Autodesk Inventor part; units mm, degrees
ref_plane "YZ Plane" through (0, 0, 0) normal (1, 0, 0) x (0, 1, 0)
ref_plane "XZ Plane" through (0, 0, 0) normal (0, 1, 0) x (-1, 0, 0)
ref_plane "XY Plane" through (0, 0, 0) normal (0, 0, 1) x (1, 0, 0)
sketch "スケッチ1" plane through (0, 0, 0) normal (0, 1, 0) x (-1, 0, 0)
  line L0 (0, 0) -> (-1.1547, 0)
  line L1 (-2.6, 1.05) -> (-3.5, 1.05)
  line L2 (-3.5, 1.05) -> (-3.5, 1.65)
  line L3 (-3.5, 1.65) -> (-1.5, 1.65)
  line L4 (-1.5, 1.65) -> (-1.5, 7.65)
  line L5 (-1.5, 7.65) -> (0, 7.65)
  line L6 (0, 7.65) -> (0, 0)
  arc A0 (-2.6, 1.05) -> (-1.1547, 0) centre (-1.1547, 1.5197) ccw
  dimension "d0" = 5.2
  dimension "d1" = 7
  dimension "d3" = 1.65
  dimension "d4" = 0.6
  dimension "d5" = 2.3094
  dimension "d6" = 6
  dimension "d7" = 3
revolve "回転1" add sketch "スケッチ1" angle 360 about axis through (0, 0, 7.65) along (0, 0, -1)
thread "ねじ1"
sketch "スケッチ2" plane through (0, 0, 0) normal (0, 0, -1) x (-1, 0, 0)
  circle A0 centre (0, 0) radius 1.1547
  line L0 (0, 1.1547) -> (1, 0.5774)
  line L1 (1, 0.5774) -> (1, -0.5774)
  line L2 (1, -0.5774) -> (0, -1.1547)
  line L3 (0, -1.1547) -> (-1, -0.5774)
  line L4 (-1, -0.5774) -> (-1, 0.5774)
  line L5 (-1, 0.5774) -> (0, 1.1547)
  point P0 (0, 0)
  point P1 (0, 0)
extrude "押し出し1" cut sketch "スケッチ2" against normal blind 1.05 contours L1 L2 L3 L4 L5 L0
properties part number "620103006" material "ステンレス鋼 AISI 304"
The model under review builds one solid part; all positions refer to its coordinate system, in mm. A direction names the side the tool comes from. Round coordinates to 2 decimals unless told otherwise and drop trailing zeros. Loops run counter-clockwise (first coordinate to the right, second up) from the corner with the lowest first, then second, coordinate; pieces in that order, holes last.
1) Consider section A-A on z = 6.5. State the section outline as (x, y) points, then the cut area to 3 significant figures.
Values follow:
outline: circle Ø3 at (0, 0)
area: 7.07 mm2
2) Tool access review of faces 4 (the face through (-0.49, 0.87, 0.52)), 5 (the face through (3.233, -1.341, 1.354)), 6 (the face through (0, 2, 1.65)): name each direction out of +Z, -Z, +X, -X, +Y, -Y from which nothing blocks a thin tool from reaching the whole face with its end or side.
Values follow:
face 4: -Z
face 5: +Z, -Z
face 6: +Z
3) Wall thickness on line 1 along Z through (x, y) = (1.75, 3); line 2 along Z through (x, y) = (0.25, -2.5); line 3 along Y through (x, z) = (-3, 1.5): over which ranges is each line inside the solid? List them lowest first.
Values follow:
line 1: z = 1.05 to 1.65
line 2: z = 0.84 to 1.65
line 3: y = -1.8 to 1.8
4) Clearance check with flat-ended pins moving along their axes: P1, Ø2, axis at x = -2, y = -0.5, coming from the -Z side; P2, Ø1.5, axis at y = 1, z = 1, coming from the +X side; P3, Ø0.5, axis at y = 0, z = 0.5, coming from the -X side; P4, Ø0.8, axis at y = 0, z = 0.5, coming from the +X side. State where each tip first meets the part, or that it passes through.
Values follow:
P1: stops at z = 0
P2: stops at x = 3.49
P3: stops at x = -2.47
P4: stops at x = 2.54
5) The part is to be moulded in two halves that separate along X. For faces 1 (the face through (-1.5, 0.07, 4.69)), 2 (the face through (0, 0, 7.65)), 3 (the face through (0, 0, 1.05)), say which applies: pulls with the +X half, pulls with the -X half, needs draft (parallel to the pull), parting line crosses it, or undercut.
Values follow:
face 1: parting line crosses it
face 2: needs draft
face 3: undercut
6) Consider section B-B on y = -3. State the section outline as (x, z) points, then the cut area to 3 significant figures.
Values follow:
outline: (-1.8, 1.05) - (1.8, 1.05) - (1.8, 1.65) - (-1.8, 1.65) - close
area: 2.16 mm2
